The listing builds one solid part. Answer for the finished solid, in the listing's coordinates (mm). Face numbers are marked on the shaded views. Round coordinates to 2 decimals unless told otherwise and drop trailing zeros. Order: outer loops, then holes, each group sorted by start corner. A loop starts at its lowest first (then second) coordinate and runs counter-clockwise, first axis right, second up. Notation, with made-up numbers: (22.25, -5.75) - (29.25, -5.75) arc R15 cw to (29.25, 9.25) - close; hole circle Ø11 at (0, 34). An arc over 180 degrees is marked (long way). Write item = value, one per line.
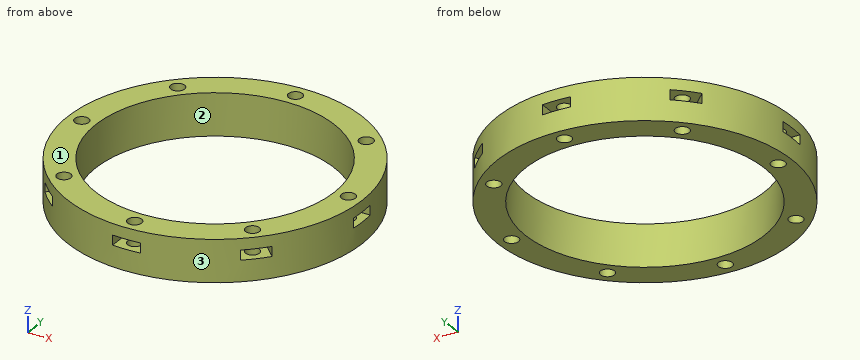
from build123d import *

# Parameters (mm, degrees)
CYLINDER2767_R               = 1
CYLINDER2767_DEPTH           = 10
CYLINDER2767_PLACEMENT_ANGLE = 45
CYLINDER2768_R               = 1
CYLINDER2768_DEPTH           = 10
CYLINDER2769_R               = 1
CYLINDER2769_DEPTH           = 10
CYLINDER2769_PLACEMENT_ANGLE = 135
CYLINDER2770_R               = 1
CYLINDER2770_DEPTH           = 10
CYLINDER2771_R               = 1
CYLINDER2771_DEPTH           = 10
CYLINDER2771_PLACEMENT_ANGLE = 225
CYLINDER2772_R               = 1
CYLINDER2772_DEPTH           = 10
CYLINDER2773_R               = 1
CYLINDER2773_DEPTH           = 10
CYLINDER2773_PLACEMENT_ANGLE = 45
CYLINDER2766_R               = 1
CYLINDER2766_DEPTH           = 10
BOX961_W                     = 4
BOX961_H                     = 4
BOX961_DEPTH                 = 1.4
BOX961_PLACEMENT_ANGLE       = 45
BOX964_W                     = 4
BOX964_H                     = 4
BOX964_DEPTH                 = 1.4
BOX962_W                     = 4
BOX962_H                     = 4
BOX962_DEPTH                 = 1.4
BOX962_PLACEMENT_ANGLE       = 135
BOX963_W                     = 4
BOX963_H                     = 4
BOX963_DEPTH                 = 1.4
BOX965_W                     = 4
BOX965_H                     = 4
BOX965_DEPTH                 = 1.4
BOX965_PLACEMENT_ANGLE       = 225
BOX967_W                     = 4
BOX967_H                     = 4
BOX967_DEPTH                 = 1.4
BOX966_W                     = 4
BOX966_H                     = 4
BOX966_DEPTH                 = 1.4
BOX966_PLACEMENT_ANGLE       = 45
BOX960_W                     = 4
BOX960_H                     = 4
BOX960_DEPTH                 = 1.4
TUBE135_R                    = 21
TUBE135_R_2                  = 17
TUBE135_DEPTH                = 6


with BuildPart() as obj1:
    # Cylinder2767 → Cylinder2767 (new body)
    with BuildSketch(Plane.XY):
        Circle(CYLINDER2767_R)
    extrude(amount=CYLINDER2767_DEPTH)


with BuildPart() as obj1_1:
    # Cylinder2767 placement: moved
    add(obj1.part.moved(Location((-13.435029, 13.435029, -20))).rotate(Axis((-13.435029, 13.435029, -20), (0, 0, 1)), CYLINDER2767_PLACEMENT_ANGLE))


with BuildPart() as obj2:
    # Cylinder2768 → Cylinder2768 (new body)
    with BuildSketch(Plane(origin=(-19, 0, -20), x_dir=(0, 1, 0), z_dir=(0, 0, 1))):
        Circle(CYLINDER2768_R)
    extrude(amount=CYLINDER2768_DEPTH)


with BuildPart() as obj3:
    # Cylinder2769 → Cylinder2769 (new body)
    with BuildSketch(Plane.XY):
        Circle(CYLINDER2769_R)
    extrude(amount=CYLINDER2769_DEPTH)


with BuildPart() as obj3_1:
    # Cylinder2769 placement: moved
    add(obj3.part.moved(Location((-13.435029, -13.435029, -20))).rotate(Axis((-13.435029, -13.435029, -20), (0, 0, 1)), CYLINDER2769_PLACEMENT_ANGLE))


with BuildPart() as obj4:
    # Cylinder2770 → Cylinder2770 (new body)
    with BuildSketch(Plane(origin=(0, -19, -20), x_dir=(-1, 0, 0), z_dir=(0, 0, 1))):
        Circle(CYLINDER2770_R)
    extrude(amount=CYLINDER2770_DEPTH)


with BuildPart() as obj5:
    # Cylinder2771 → Cylinder2771 (new body)
    with BuildSketch(Plane.XY):
        Circle(CYLINDER2771_R)
    extrude(amount=CYLINDER2771_DEPTH)


with BuildPart() as obj5_1:
    # Cylinder2771 placement: moved
    add(obj5.part.moved(Location((13.435029, -13.435029, -20))).rotate(Axis((13.435029, -13.435029, -20), (0, 0, 1)), CYLINDER2771_PLACEMENT_ANGLE))


with BuildPart() as obj6:
    # Cylinder2772 → Cylinder2772 (new body)
    with BuildSketch(Plane(origin=(19, 0, -20), x_dir=(0, -1, 0), z_dir=(0, 0, 1))):
        Circle(CYLINDER2772_R)
    extrude(amount=CYLINDER2772_DEPTH)


with BuildPart() as obj7:
    # Cylinder2773 → Cylinder2773 (new body)
    with BuildSketch(Plane.XY):
        Circle(CYLINDER2773_R)
    extrude(amount=CYLINDER2773_DEPTH)


with BuildPart() as obj7_1:
    # Cylinder2773 placement: moved
    add(obj7.part.moved(Location((13.435029, 13.435029, -20))).rotate(Axis((13.435029, 13.435029, -20), (0, 0, -1)), CYLINDER2773_PLACEMENT_ANGLE))


with BuildPart() as compound1237:
    # Cylinder2766 → Cylinder2766 (new body)
    with BuildSketch(Plane(origin=(0, 19, -20), x_dir=(1, 0, 0), z_dir=(0, 0, 1))):
        Circle(CYLINDER2766_R)
    extrude(amount=CYLINDER2766_DEPTH)

    # Compound1237: union obj1, obj2, obj3, obj4, obj5, obj6, obj7
    add(obj1_1.part)
    add(obj2.part)
    add(obj3_1.part)
    add(obj4.part)
    add(obj5_1.part)
    add(obj6.part)
    add(obj7_1.part)


with BuildPart() as krychle960:
    # Box961 → Box961 (new body)
    with BuildSketch(Plane.XY):
        with Locations((2, 2)):
            Rectangle(BOX961_W, BOX961_H)
    extrude(amount=BOX961_DEPTH)


with BuildPart() as krychle960_1:
    # Box961 placement: moved
    add(krychle960.part.moved(Location((-13.435029, 10.606602, -13))).rotate(Axis((-13.435029, 10.606602, -13), (0, 0, 1)), BOX961_PLACEMENT_ANGLE))


with BuildPart() as krychle963:
    # Box964 → Box964 (new body)
    with BuildSketch(Plane(origin=(-17, -2, -13), x_dir=(0, 1, 0), z_dir=(0, 0, 1))):
        with Locations((2, 2)):
            Rectangle(BOX964_W, BOX964_H)
    extrude(amount=BOX964_DEPTH)


with BuildPart() as krychle961:
    # Box962 → Box962 (new body)
    with BuildSketch(Plane.XY):
        with Locations((2, 2)):
            Rectangle(BOX962_W, BOX962_H)
    extrude(amount=BOX962_DEPTH)


with BuildPart() as krychle961_1:
    # Box962 placement: moved
    add(krychle961.part.moved(Location((-10.606602, -13.435029, -13))).rotate(Axis((-10.606602, -13.435029, -13), (0, 0, 1)), BOX962_PLACEMENT_ANGLE))


with BuildPart() as krychle962:
    # Box963 → Box963 (new body)
    with BuildSketch(Plane(origin=(2, -17, -13), x_dir=(-1, 0, 0), z_dir=(0, 0, 1))):
        with Locations((2, 2)):
            Rectangle(BOX963_W, BOX963_H)
    extrude(amount=BOX963_DEPTH)


with BuildPart() as krychle964:
    # Box965 → Box965 (new body)
    with BuildSketch(Plane.XY):
        with Locations((2, 2)):
            Rectangle(BOX965_W, BOX965_H)
    extrude(amount=BOX965_DEPTH)


with BuildPart() as krychle964_1:
    # Box965 placement: moved
    add(krychle964.part.moved(Location((13.435029, -10.606602, -13))).rotate(Axis((13.435029, -10.606602, -13), (0, 0, 1)), BOX965_PLACEMENT_ANGLE))


with BuildPart() as krychle966:
    # Box967 → Box967 (new body)
    with BuildSketch(Plane(origin=(17, 2, -13), x_dir=(0, -1, 0), z_dir=(0, 0, 1))):
        with Locations((2, 2)):
            Rectangle(BOX967_W, BOX967_H)
    extrude(amount=BOX967_DEPTH)


with BuildPart() as krychle965:
    # Box966 → Box966 (new body)
    with BuildSketch(Plane.XY):
        with Locations((2, 2)):
            Rectangle(BOX966_W, BOX966_H)
    extrude(amount=BOX966_DEPTH)


with BuildPart() as krychle965_1:
    # Box966 placement: moved
    add(krychle965.part.moved(Location((10.606602, 13.435029, -13))).rotate(Axis((10.606602, 13.435029, -13), (0, 0, -1)), BOX966_PLACEMENT_ANGLE))


with BuildPart() as compound1236:
    # Box960 → Box960 (new body)
    with BuildSketch(Plane(origin=(-2, 17, -13), x_dir=(1, 0, 0), z_dir=(0, 0, 1))):
        with Locations((2, 2)):
            Rectangle(BOX960_W, BOX960_H)
    extrude(amount=BOX960_DEPTH)

    # Compound1236: union Krychle960, Krychle963, Krychle961, Krychle962, Krychle964, Krychle966, Krychle965
    add(krychle960_1.part)
    add(krychle963.part)
    add(krychle961_1.part)
    add(krychle962.part)
    add(krychle964_1.part)
    add(krychle966.part)
    add(krychle965_1.part)


with BuildPart() as cut1045:
    # Tube135 → Tube135 (new body)
    with BuildSketch(Plane.XY.offset(-16)):
        Circle(TUBE135_R)
        Circle(TUBE135_R_2, mode=Mode.SUBTRACT)
    extrude(amount=TUBE135_DEPTH)

    # Cut1044: cut Compound1236
    add(compound1236.part, mode=Mode.SUBTRACT)

    # Cut1045: cut Compound1237
    add(compound1237.part, mode=Mode.SUBTRACT)


solid = cut1045.part
Q1. Find the intervals of material crossed by line 1 (X direction, y = 0, z = -11.3); line 2 (Z direction, x = 0, y = -17.5); line 3 (Y direction, x = 3, z = -10.7), in increasing order. Write a range as from..to.
Model answer:
line_1 = -21..-20, -18..-17, 17..18, 20..21
line_2 = -16..-13, -11.6..-10
line_3 = -20.78..-16.73, 16.73..20.78
Q2. Section A-A on y = -19 is taken. Determine the outline of the cut face in (x, z).
Model answer:
outline = (-8.94, -16) - (-1, -16) - (-1, -13) - (-2, -13) - (-2, -11.6) - (-1, -11.6) - (-1, -10) - (-8.94, -10) - close; (1, -16) - (8.94, -16) - (8.94, -10) - (1, -10) - (1, -11.6) - (2, -11.6) - (2, -13) - (1, -13) - close
Q3. Determine the mould class of the marked faces 1, 2 and 3 for opening direction X: released by +X, released by -X, zero draft, split by the parting line, or undercut.
Model answer:
face_1 = zero draft
face_2 = undercut
face_3 = split by the parting line
Q4. Section C-C on x = 3 is taken. Determine the outline of the cut face in (y, z), then the cut area to 3 significant figures.
Model answer:
outline = (-20.78, -16) - (-16.73, -16) - (-16.73, -10) - (-20.78, -10) - close; (16.73, -16) - (20.78, -16) - (20.78, -10) - (16.73, -10) - close
area = 48.6 mm^2
Q5. Section D-D on y = -2.5 is taken. Determine the outline of the cut face in (x, z), then the cut area to 3 significant figures.
Model answer:
outline = (-20.85, -16) - (-16.82, -16) - (-16.82, -10) - (-20.85, -10) - close; (16.82, -16) - (20.85, -16) - (20.85, -10) - (16.82, -10) - close
area = 48.4 mm^2
Q6. Flat-ended cylindrical pins translate along their axes: P1, Ø3, axis at y = 3.5, z = -15, coming from the +X side; P2, Ø0.7, axis at y = 19.5, z = -12.5, coming from the -X side; P3, Ø1.5, axis at x = 1, z = -12.5, coming from the -Y side; P4, Ø1.8, axis at x = -19, y = 0, coming from the -Z side. Find the tip coordinate at first contact, or state that the pin passes through.
Model answer:
P1 = 20.9
P2 = -8.62
P3 = -21
P4 = through
Q7. Section B-B on z = -14.95 is taken. Count the separate pieces of the cut face and the enclosed holes in it, then the cut area to 3 significant figures.
Model answer:
separate_pieces = 1
enclosed_holes = 9
area = 452 mm^2
